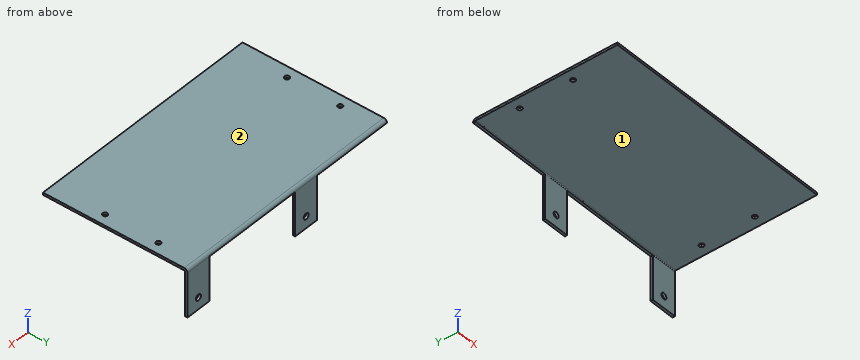
```python
from build123d import *

# Parameters (mm, degrees)
SKETCH2_W                    = 200
SKETCH2_H                    = 120
BASE_FLANGE1_DEPTH           = 2
CUT_EXTRUDE1_REACH           = 235.247
SKETCH7_R                    = 2
EDGE_FLANGE1_STRIP_W         = 9.4732
EDGE_FLANGE1_STRIP_H         = 2
EDGE_FLANGE1_STRIP_CUT_DEPTH = 200
EDGE_FLANGE1_DEPTH           = 200
CUT_EXTRUDE2_REACH           = 239.664
SKETCH11_R                   = 2.5
SKETCH11_W                   = 86
SKETCH11_H                   = 37.2634
SKETCH11_W_2                 = 70


# Sheet-metal steps are written as plain solids
with BuildPart() as part:
    # Sketch2 → Base-Flange1 (new body)
    with BuildSketch(Plane.XY):
        with Locations((100, 60)):
            Rectangle(SKETCH2_W, SKETCH2_H)
    extrude(amount=-BASE_FLANGE1_DEPTH)

    # Sketch7 → Cut-Extrude1 (cut, up to next)
    with BuildSketch(Plane.XY, mode=Mode.PRIVATE) as cut_extrude1_sk1:
        with Locations((8.87, 90)):
            Circle(SKETCH7_R)
    cut_extrude1_tool1 = extrude(cut_extrude1_sk1.sketch, amount=-CUT_EXTRUDE1_REACH, mode=Mode.PRIVATE) & part.part
    # Sketch7 → Cut-Extrude1 (cut, up to next)
    with BuildSketch(Plane.XY, mode=Mode.PRIVATE) as cut_extrude1_sk2:
        with Locations((8.87, 45)):
            Circle(SKETCH7_R)
    cut_extrude1_tool2 = extrude(cut_extrude1_sk2.sketch, amount=-CUT_EXTRUDE1_REACH, mode=Mode.PRIVATE) & part.part
    # Sketch7 → Cut-Extrude1 (cut, up to next)
    with BuildSketch(Plane.XY, mode=Mode.PRIVATE) as cut_extrude1_sk3:
        with Locations((191.13, 45)):
            Circle(SKETCH7_R)
    cut_extrude1_tool3 = extrude(cut_extrude1_sk3.sketch, amount=-CUT_EXTRUDE1_REACH, mode=Mode.PRIVATE) & part.part
    # Sketch7 → Cut-Extrude1 (cut, up to next)
    with BuildSketch(Plane.XY, mode=Mode.PRIVATE) as cut_extrude1_sk4:
        with Locations((191.13, 90)):
            Circle(SKETCH7_R)
    cut_extrude1_tool4 = extrude(cut_extrude1_sk4.sketch, amount=-CUT_EXTRUDE1_REACH, mode=Mode.PRIVATE) & part.part
    add(cut_extrude1_tool1.solids().sort_by_distance((8.87, 90, 0))[0], mode=Mode.SUBTRACT)
    add(cut_extrude1_tool2.solids().sort_by_distance((8.87, 45, 0))[0], mode=Mode.SUBTRACT)
    add(cut_extrude1_tool3.solids().sort_by_distance((191.13, 45, 0))[0], mode=Mode.SUBTRACT)
    add(cut_extrude1_tool4.solids().sort_by_distance((191.13, 90, 0))[0], mode=Mode.SUBTRACT)

    # Edge-Flange1 strip (across the edge) → Edge-Flange1 strip cut (cut)
    with BuildSketch(Plane(origin=(0, 120, -2), x_dir=(0, -1, 0), z_dir=(1, 0, 0))):
        with Locations((-4, -1)):
            Rectangle(EDGE_FLANGE1_STRIP_W, EDGE_FLANGE1_STRIP_H)
    extrude(amount=EDGE_FLANGE1_STRIP_CUT_DEPTH, mode=Mode.SUBTRACT)

    # Edge-Flange1 section (across the edge) → Edge-Flange1 (add)
    with BuildSketch(Plane(origin=(0, 120, -2), x_dir=(0, -1, 0), z_dir=(1, 0, 0))):
        with BuildLine():
            Line((-2, 0.7366), (-2, 38))
            Line((-2, 38), (0, 38))
            Line((0, 38), (0, 0.7366))
            ThreePointArc((0, 0.7366), (0.215745145, 0.215745145), (0.7366, 0))
            Line((0.7366, 0), (0.7366, -2))
            ThreePointArc((0.7366, -2), (-1.198468417, -1.198468417), (-2, 0.7366))
        make_face()
    extrude(amount=EDGE_FLANGE1_DEPTH)

    # Sketch11 → Cut-Extrude2 (cut, up to next)
    with BuildSketch(Plane(origin=(0, 122, 0), x_dir=(1, 0, 0), z_dir=(0, 1, 0)), mode=Mode.PRIVATE) as cut_extrude2_sk1:
        with Locations(Location((189, 30, 0), (0, 0, 270))):
            Circle(SKETCH11_R)
    cut_extrude2_tool1 = extrude(cut_extrude2_sk1.sketch, amount=-CUT_EXTRUDE2_REACH, mode=Mode.PRIVATE) & part.part
    # Sketch11 → Cut-Extrude2 (cut, up to next)
    with BuildSketch(Plane(origin=(0, 122, 0), x_dir=(1, 0, 0), z_dir=(0, 1, 0)), mode=Mode.PRIVATE) as cut_extrude2_sk2:
        with Locations(Location((81, 30, 0), (0, 0, 270))):
            Circle(SKETCH11_R)
    cut_extrude2_tool2 = extrude(cut_extrude2_sk2.sketch, amount=-CUT_EXTRUDE2_REACH, mode=Mode.PRIVATE) & part.part
    # Sketch11 → Cut-Extrude2 (cut, up to next)
    with BuildSketch(Plane(origin=(0, 122, 0), x_dir=(1, 0, 0), z_dir=(0, 1, 0)), mode=Mode.PRIVATE) as cut_extrude2_sk3:
        with Locations((135, 21.3683)):
            Rectangle(SKETCH11_W, SKETCH11_H)
    cut_extrude2_tool3 = extrude(cut_extrude2_sk3.sketch, amount=-CUT_EXTRUDE2_REACH, mode=Mode.PRIVATE) & part.part
    # Sketch11 → Cut-Extrude2 (cut, up to next)
    with BuildSketch(Plane(origin=(0, 122, 0), x_dir=(1, 0, 0), z_dir=(0, 1, 0)), mode=Mode.PRIVATE) as cut_extrude2_sk4:
        with Locations((35, 21.3683)):
            Rectangle(SKETCH11_W_2, SKETCH11_H)
    cut_extrude2_tool4 = extrude(cut_extrude2_sk4.sketch, amount=-CUT_EXTRUDE2_REACH, mode=Mode.PRIVATE) & part.part
    add(cut_extrude2_tool1.solids().sort_by_distance((189, 122, -30))[0], mode=Mode.SUBTRACT)
    add(cut_extrude2_tool2.solids().sort_by_distance((81, 122, -30))[0], mode=Mode.SUBTRACT)
    add(cut_extrude2_tool3.solids().sort_by_distance((135, 122, -21.3683))[0], mode=Mode.SUBTRACT)
    add(cut_extrude2_tool4.solids().sort_by_distance((35, 122, -21.3683))[0], mode=Mode.SUBTRACT)


solid = part.part
```
Work out the finished part from the listing and answer in its coordinate system (mm). Face numbers are marked on the shaded views. A direction names the side the tool comes from. Give positions to 0.01 mm unless a question says otherwise; leave off trailing zeros. Order: outer loops, then holes, each group sorted by start corner. A loop starts at its lowest first (then second) coordinate and runs counter-clockwise, first axis right, second up.
1. For the marked faces 1 and 2, determine the directions among +Z, -Z, +X, -X, +Y, -Y from which every point of the face is accessible in a straight line to the end or side of a thin tool.
Result sheet:
face 1: -Z, +X, -X, -Y
face 2: +Z, +X, -X, +Y, -Y
2. Section B-B, the plane x = 8.87 is taken. Determine the outline of the cut face in (y, z).
Result sheet:
outline: (0, -2) - (43, -2) - (43, 0) - (0, 0) - close; (47, -2) - (88, -2) - (88, 0) - (47, 0) - close; (92, -2) - (119.26, -2) arc R0.74 cw to (120, -2.74) - (122, -2.74) arc R2.74 ccw to (119.26, 0) - (92, 0) - close
3. Section D-D, the plane x = 81 is taken. Determine the outline of the cut face in (y, z).
Result sheet:
outline: (0, -2) - (119.26, -2) arc R0.74 cw to (120, -2.74) - (120, -27.5) - (122, -27.5) - (122, -2.74) arc R2.74 ccw to (119.26, 0) - (0, 0) - close; (120, -40) - (122, -40) - (122, -32.5) - (120, -32.5) - close
4. Each of these flat-tipped pins is pushed along its axis until it touches: P1, Ø12, axis at y = 70.5, z = -13, coming from the -X side; P2, Ø5, axis at x = 191.13, y = 45, coming from the -Z side; P3, Ø1, axis at y = 120.5, z = -19.5, coming from the -X side; P4, Ø17.5, axis at x = 82, z = -21.5, coming from the -Y side. Where does it stop, or does it pass through?
Result sheet:
P1: passes through
P2: stops at z = -2
P3: stops at x = 70
P4: stops at y = 120
5. Section A-A, the plane y = 90 is taken. Determine the outline of the cut face in (x, z), and give its area (3 significant figures).
Result sheet:
outline: (0, -2) - (6.87, -2) - (6.87, 0) - (0, 0) - close; (10.87, -2) - (189.13, -2) - (189.13, 0) - (10.87, 0) - close; (193.13, -2) - (200, -2) - (200, 0) - (193.13, 0) - close
area: 384 mm2
6. Straight lines are drawn through the part: L1, parallel to X at y = 121.15, z = -30; L2, parallel to Y at x = 191.13, z = -1.15; L3, parallel to Y at x = 191.13, z = -0.8. For each, find the intervals that lie inside material, in ascending order.
Result sheet:
L1: x = 70 to 78.5, 83.5 to 92, 178 to 186.5, 191.5 to 200
L2: y = 0 to 43, 47 to 88, 92 to 121.49
L3: y = 0 to 43, 47 to 88, 92 to 121.2
7. Section C-C, the plane z = -23 is taken. Determine the outline of the cut face in (x, y), and give its area (3 significant figures).
Result sheet:
outline: (70, 120) - (92, 120) - (92, 122) - (70, 122) - close; (178, 120) - (200, 120) - (200, 122) - (178, 122) - close
area: 88.0 mm2
